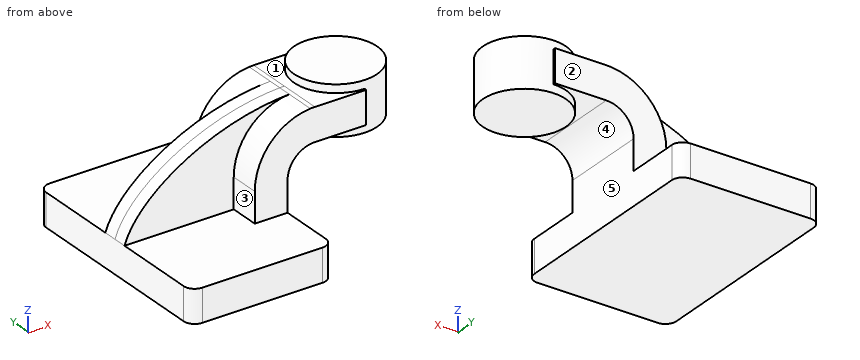
from build123d import *

# Parameters (mm, degrees)
F1_DEPTH = 63.5
F0_W     = 26.6420548012
F0_H     = 19.05
F2_DEPTH = 25.4
F3_DEPTH = 7.9375
F5_R     = 6.35


# Not quite as in the source:
# - a feature of the source that left no trace in its solid (it failed there, or was rolled back) is left out


with BuildPart() as f1:
    # F0 (on Front) → F1 (new body, symmetric)
    with BuildSketch(Plane.XZ):
        Polygon((-41.275, 9.525), (-41.275, -9.525), (41.275, -9.525), (41.275, 9.525), (22.225, 9.525), align=None)
    extrude(amount=F1_DEPTH, both=True)

    # F0 (on Front) → F2 (join, symmetric)
    with BuildSketch(Plane.XZ):
        with BuildLine():
            Line((22.225, 9.525), (41.275, 9.525))
            Line((41.275, 9.525), (41.275, 27.0002))
            ThreePointArc((41.275, 27.0002), (45.9246798487, 38.2255201513), (57.15, 42.8752))
            Line((57.15, 42.8752), (60.325, 42.8752))
            Line((60.325, 42.8752), (60.325, 61.9252))
            Line((60.325, 61.9252), (57.15, 61.9252))
            add(Edge.make_bspline(
                [(54.5213953348, 61.8261395066), (55.3958874756, 61.867746875), (56.2721525992, 61.9008262266), (57.15, 61.9252)],
                knots=[109.4468822065, 109.4468822065, 109.4468822065, 109.4468822065, 111.5045361635, 111.5045361635, 111.5045361635, 111.5045361635], degree=3))
            ThreePointArc((54.5213953348, 61.8261395066), (31.5418016747, 50.7483747411), (22.225, 27.0002))
            Line((22.225, 27.0002), (22.225, 9.525))
        make_face()
        with Locations((73.6460274006, 52.4002)):
            Rectangle(F0_W, F0_H)
    extrude(amount=F2_DEPTH, both=True)

    # F0 (on Front) → F3 (join, symmetric)
    with BuildSketch(Plane.XZ):
        with BuildLine():
            add(Edge.make_bspline(
                [(-41.275, 9.525), (-33.4912011652, 33.272556952), (8.0070443726, 59.6130381539), (54.5213953348, 61.8261395066)],
                knots=[0, 0, 0, 0, 109.4468822065, 109.4468822065, 109.4468822065, 109.4468822065], degree=3))
            Line((-41.275, 9.525), (22.225, 9.525))
            Line((22.225, 9.525), (22.225, 27.0002))
            ThreePointArc((22.225, 27.0002), (31.5418016747, 50.7483747411), (54.5213953348, 61.8261395066))
        make_face()
    extrude(amount=F3_DEPTH, both=True)

    # F0 (on Front) → F4 (revolve)
    with BuildSketch(Plane.XZ):
        Polygon((86.9670548012, 66.675), (86.9670548012, 61.9252), (86.9670548012, 42.8752), (86.9670548012, 38.1), (111.125, 38.1), (111.125, 66.675), align=None)
    revolve(axis=Axis((86.9670548012, 0, 52.3875), (0, 0, 1)))

    # F5
    f5_edges = [f1.edges().sort_by_distance(p)[0] for p in [
        (-41.275, -63.5, 0),
        (41.275, -63.5, 0),
        (41.275, 63.5, 0),
        (-41.275, 63.5, 0),
    ]]
    fillet(f5_edges, radius=F5_R)


solid = f1.part
Geometry check sheet. Reference: the model listing, model coordinates, mm. Face numbers are marked on the shaded views. A direction names the side the tool comes from. Round coordinates to 2 decimals unless told otherwise and drop trailing zeros. Order: outer loops, then holes, each group sorted by start corner. A loop starts at its lowest first (then second) coordinate and runs counter-clockwise, first axis right, second up. Notation, with made-up numbers: M -9,23 L 11,23 A15 cw 11,35 Z; hole C 82,-0.5 d8. An arc over 180 degrees is marked long. Write each question's results on one line, items separated by ' | '. Start each with the question number.
1. Go/stop test with flat-tipped pins: P1, Ø16.5, axis at x = -12.5, y = 25, coming from the +Z side (3 decimals); P2, Ø3, axis at y = 18, z = 45, coming from the -X side; P3, Ø24, axis at x = 83, y = -1, coming from the -Z side. Record where each tip stops, or that it passes through.
2. Cross-section at A-A on x = 72. Record the boundary of the cut face in (y, z) (3 decimals).
3. Material ranges on L1, parallel to Y at x = 36.5, z = 37.5; L2, parallel to Z at x = 14.5, y = 8.5 (3 decimals); L3, parallel to X at y = 26.5, z = -0.5 (3 decimals), recorded low to high. Write a range as from..to.
4. Cross-section at B-B on y = 52. Record the boundary of the cut face in (x, z) (3 decimals), plus the area to 3 significant figures.
5. Set-up check for the marked faces 1, 2, 3, 4 and 5: record each of +Z, -Z, +X, -X, +Y, -Y from which the full face is reachable in a straight line by a thin tool's end or side.
Resolved:
1) P1: z = 9.525 | P2: x = 26.37 | P3: z = 38.1
2) outline: M -25.4,42.875 L -18.963,42.875 L -18.963,38.1 L 18.963,38.1 L 18.963,42.875 L 25.4,42.875 L 25.4,61.925 L 18.963,61.925 L 18.963,66.675 L -18.963,66.675 L -18.963,61.925 L -25.4,61.925 Z
3) L1: -25.4..25.4 | L2: -9.525..9.525 | L3: -41.275..41.275
4) outline: M -41.275,-9.525 L 41.275,-9.525 L 41.275,9.525 L -41.275,9.525 Z | area: 1,570 mm2
5) face 1: +Z, -X | face 2: +Z, +X, -X, +Y | face 3: +Z, -X, -Y | face 4: -Z, +Y, -Y | face 5: -Z, +X, +Y, -Y
